```python
from build123d import *

# Parameters (mm, degrees)
F1_DEPTH = 127
F2_R     = 38.1


with BuildPart() as f1:
    # F0 (on Top) → F1 (new body)
    with BuildSketch(Plane.XY):
        Polygon((470.323251, 669.416738), (-444.076749, 669.416738), (-444.076749, -346.583262), (-291.676749, -346.583262), (-291.676749, -257.683262), (-355.176749, -257.683262), (-355.176749, 580.516738), (381.423251, 580.516738), (381.423251, -257.683262), (317.923251, -257.683262), (317.923251, -346.583262), (470.323251, -346.583262), align=None)
    extrude(amount=F1_DEPTH)

    # F2
    f2_edges = [f1.edges().sort_by_distance(p)[0] for p in [
        (13.123251, 669.416738, 0),
        (13.123251, 669.416738, 127),
        (470.323251, 161.416738, 127),
        (470.323251, 161.416738, 0),
        (-444.076749, 161.416738, 0),
        (-444.076749, 161.416738, 127),
        (-367.876749, -346.583262, 0),
        (-367.876749, -346.583262, 127),
        (394.123251, -346.583262, 127),
        (394.123251, -346.583262, 0),
    ]]
    fillet(f2_edges, radius=F2_R)


solid = f1.part
```
Source: CAD feature listing. Evaluate the final solid. Frame: model axes, mm. A direction names the side the tool comes from. Round coordinates to 2 decimals unless told otherwise and drop trailing zeros. Loops run counter-clockwise (first coordinate to the right, second up) from the corner with the lowest first, then second, coordinate; pieces in that order, holes last. Notation, with made-up numbers: (79.25, 79) - (130.25, 79) arc R16 ccw to (130.25, 85) - close; hole circle Ø7 at (52.25, 5.25). An arc over 180 degrees is marked (long way). Use CSV: the item, a comma, the result in double quotes.
Q1. Section query C-C, the plane z = 57. Output: boundary loops of the cut face in (x, y), then the cut area to 3 significant figures.
Reported:
outline,"(-444.08, -346.58) - (-291.68, -346.58) - (-291.68, -257.68) - (-355.18, -257.68) - (-355.18, 580.52) - (381.42, 580.52) - (381.42, -257.68) - (317.92, -257.68) - (317.92, -346.58) - (470.32, -346.58) - (470.32, 669.42) - (-444.08, 669.42) - close"
area,"257,000 mm^2"
Q2. Reachability of faces 5 (the cylindrical face through (459.5, 168.5, 115.5)), 6 (the flat face through (381.423, 167, 63)) from +Z, -Z, +X, -X, +Y, -Y: full face, straight path, thin tool, end or side. Return the list, or none.
Reported:
face 5,"+Z, +X, +Y, -Y"
face 6,"+Z, -Z"
Q3. Ray query, line 1 along X through (y, z) = (81.5, 68); line 2 along Y through (x, z) = (-15.5, 46); line 3 along X through (y, z) = (-294.5, 34.5). Return the intervals inside material, ascending.
Reported:
line 1,"-444.08 to -355.18, 381.42 to 470.32"
line 2,"580.52 to 669.42"
line 3,"-443.91 to -291.68, 317.92 to 470.15"
Q4. Section query A-A, the plane x = -338. Output: boundary loops of the cut face in (y, z).
Reported:
outline,"(-346.58, 38.1) arc R38.1 ccw to (-308.48, 0) - (-257.68, 0) - (-257.68, 127) - (-308.48, 127) arc R38.1 ccw to (-346.58, 88.9) - close; (580.52, 0) - (631.32, 0) arc R38.1 ccw to (669.42, 38.1) - (669.42, 88.9) arc R38.1 ccw to (631.32, 127) - (580.52, 127) - close"
Q5. Mould query, pull axis X, two halves, no side actions, for faces 1 (the flat face through (20, 669.417, 63)), 2 (the flat face through (-323, -257.683, 63)), 3 (the flat face through (470.323, 154, 63)), 4 (the flat face through (317.923, -302, 63)). Classes: pulls with the +X half, pulls with the -X half, needs draft (parallel to the pull), parting line crosses it, or undercut.
Reported:
face 1,"needs draft"
face 2,"undercut"
face 3,"pulls with the +X half"
face 4,"undercut"
Q6. Section query D-D, the plane x = 151. Output: boundary loops of the cut face in (y, z), then the cut area to 3 significant figures.
Reported:
outline,"(580.52, 0) - (631.32, 0) arc R38.1 ccw to (669.42, 38.1) - (669.42, 88.9) arc R38.1 ccw to (631.32, 127) - (580.52, 127) - close"
area,"10,700 mm^2"
Q7. Section query B-B, the plane y = 132.5. Output: boundary loops of the cut face in (x, z).
Reported:
outline,"(-444.08, 38.1) arc R38.1 ccw to (-405.98, 0) - (-355.18, 0) - (-355.18, 127) - (-405.98, 127) arc R38.1 ccw to (-444.08, 88.9) - close; (381.42, 0) - (432.22, 0) arc R38.1 ccw to (470.32, 38.1) - (470.32, 88.9) arc R38.1 ccw to (432.22, 127) - (381.42, 127) - close"
Q8. Pin query (flat end, axial travel): pin 1 Ø5 at (y, z) = (-92.5, 112.5) entering from +X; pin 2 Ø12 at (y, z) = (-214, 16) entering from -X; pin 3 Ø10 at (y, z) = (260, 25) entering from -X. Return the tip coordinate at first contact, or that it passes through.
Reported:
pin 1,"x = 463.95"
pin 2,"x = -440.51"
pin 3,"x = -443.21"
